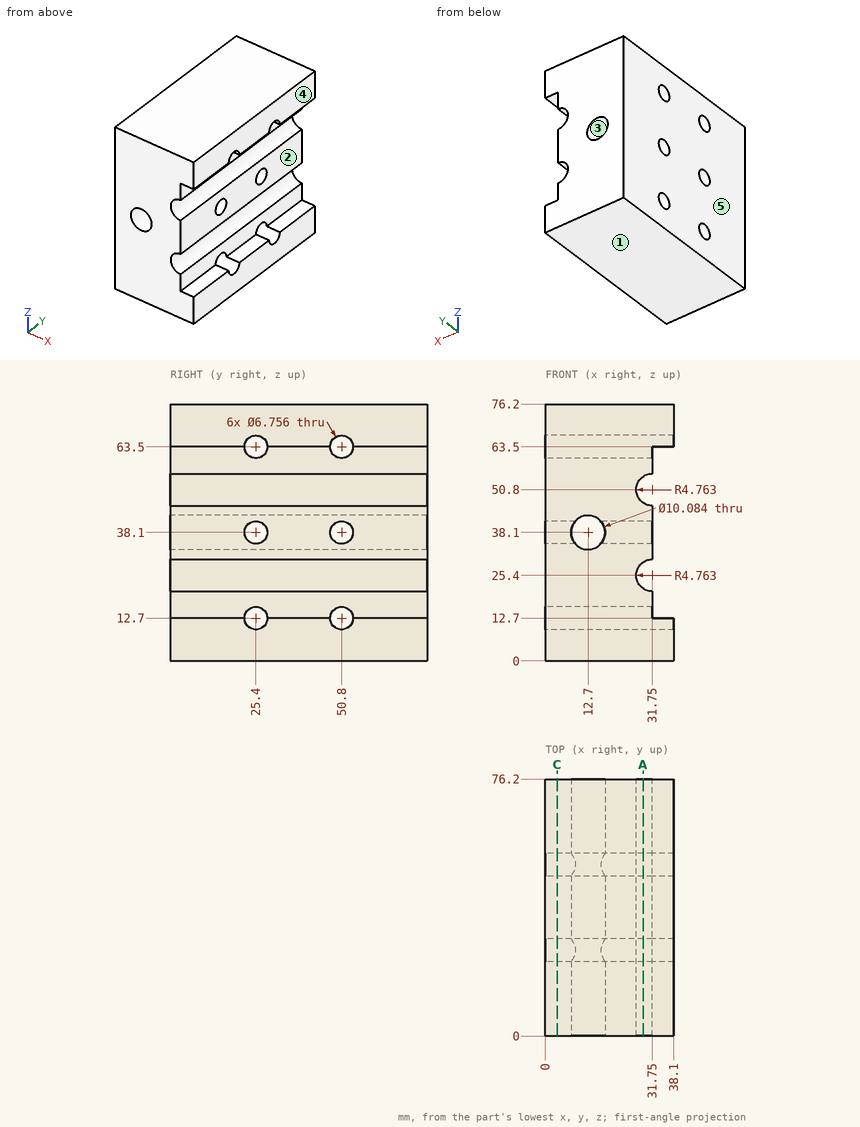
Job drawing, mm, ordinate dimensions from the low corner. One solid piece. A direction names the side the tool comes from. Round coordinates to 2 decimals unless told otherwise and drop trailing zeros. Write each loop counter-clockwise with the first axis right and the second up, starting at its lowest first coordinate (ties: lowest second). Pieces come first, ordered by that corner, then holes. Notation, with made-up numbers: M 82,-35 L 111,-35 A16 ccw 111,-24 Z; hole C 5,22.25 d10. An arc over 180 degrees is marked long. Return JSON: item names as keys, results as strings. Group by question number.
(1) Which spindle directions (+Z, -Z, +X, -X, +Y, -Y) get a long thin tool onto all of the face, cutting with end or side? Do the marked faces 1 and 2. Say none if no direction does.
(2) Pin check, flat tip, straight feed: pin 1 Ø12.5 at (y, z) = (55, 35) entering from +X. Stop position of the tip, or through.
(3) Two-plate mould, pull along X, no slides. Class the marked faces 3, 4 and 5: +X half, -X half, draft (parallel to the pull), parting line (faces both ways), or undercut.
(4) Saw through at C-C on x = 3.5. Write the cut outline in (y, z).
(5) Saw through at A-A on x = 29. Count the separate pieces of the cut face and the enclosed holes in it, then the cut area to 3 significant figures.
(6) Drill centre lines: probe 1 along Y at (x, z) = (3, 38); probe 2 along Z at (x, y) = (15, 50) (1 decimal); probe 3 along Z at (x, y) = (29, 50). Where is each one in solid material? Low to high.
Returned:
{
 "1": {"face 1": "-Z, +X, -X, +Y, -Y", "face 2": "+X, +Y, -Y"},
 "2": {"pin 1": "x = 31.75"},
 "3": {"face 3": "undercut", "face 4": "+X half", "face 5": "-X half"},
 "4": {"outline": "M 0,0 L 76.2,0 L 76.2,76.2 L 0,76.2 Z; hole C 25.4,12.7 d6.76; hole C 25.4,38.1 d6.76; hole C 25.4,63.5 d6.76; hole C 50.8,12.7 d6.76; hole C 50.8,38.1 d6.76; hole C 50.8,63.5 d6.76"},
 "5": {"separate pieces": "3", "enclosed holes": "6", "area": "4,410 mm²"},
 "6": {"probe 1": "0 to 22.02, 28.78 to 47.42, 54.18 to 76.2", "probe 2": "0 to 9.4, 16 to 33.6, 42.6 to 60.2, 66.8 to 76.2", "probe 3": "0 to 9.42, 15.98 to 21.51, 29.29 to 34.82, 41.38 to 46.91, 54.69 to 60.22, 66.78 to 76.2"}
}
